Geometry: see drawing. Coordinates: mm, zero at the bounding-box minimum. A direction names the side the tool comes from. Round coordinates to 2 decimals unless told otherwise and drop trailing zeros. Loops run counter-clockwise (first coordinate to the right, second up) from the corner with the lowest first, then second, coordinate; pieces in that order, holes last.
(1) Set-up query: the marked faces 1 and 2. Return all of +Z, -Z, +X, -X, +Y, -Y with unobstructed straight access to the full face (end or side cutting, diameter ignored); none if empty.
(2) Section B-B, the plane z = 2.45. Return the cut outline in (x, y) (1 decimal).
(3) First-contact query: pin 1 Ø1.5 at (x, z) = (10, 2) entering from +Y. Flat tip, straight axial feed; report the tip coordinate or a pass-through.
(4) Section C-C, the plane x = 3. Return the cut outline in (y, z) (1 decimal).
(5) Section A-A, the plane y = 12. Return the cut outline in (x, z) (1 decimal).
(6) Material intervals for probe 1 along X at (y, z) = (20, 0.4); probe 2 along Y at (x, z) = (3.5, 2.05) (1 decimal); probe 3 along Y at (x, z) = (2.5, 2.4) (1 decimal), sorted ascending.
(7) Mould query, pull axis X, two halves, no side actions, for the marked faces 3, 4 and 5. Classes: pulls with the +X half, pulls with the -X half, needs draft (parallel to the pull), parting line crosses it, or undercut.
(8) Section D-D, the plane x = 10.5. Return the cut outline in (y, z) (1 decimal).
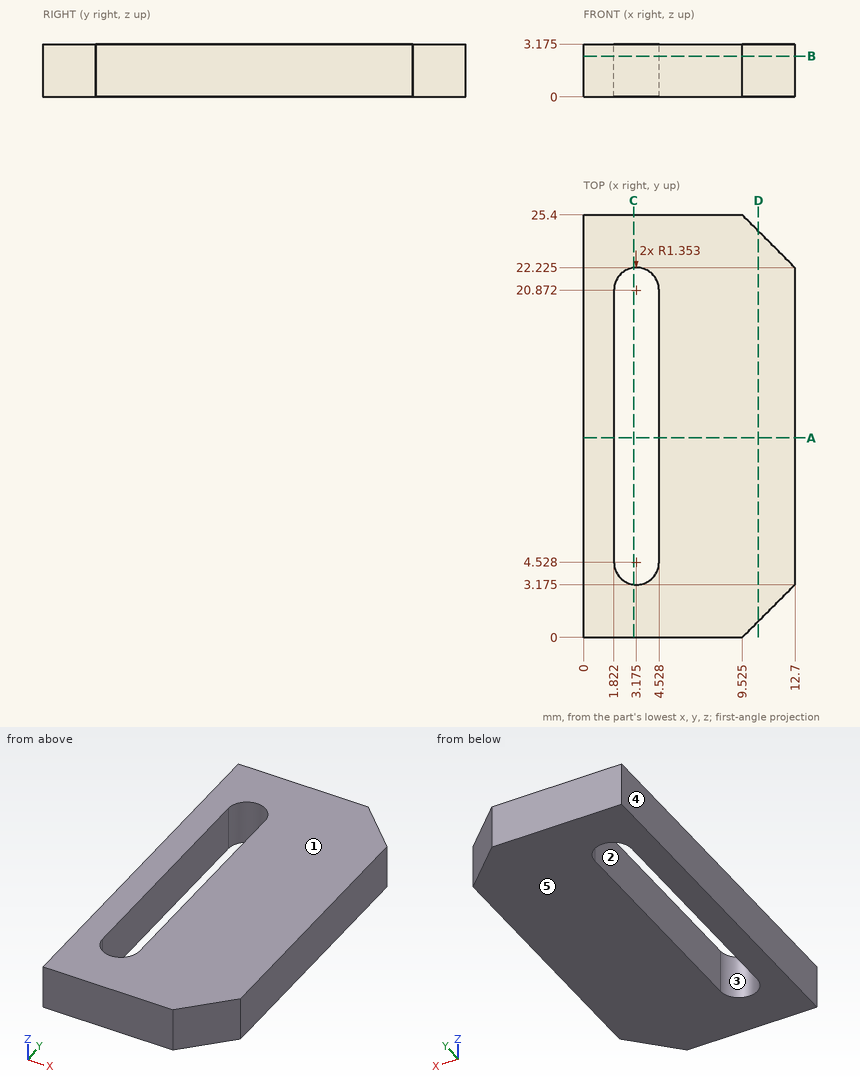
Output values:
1. face 1: +Z, +X, -X, +Y, -Y
1. face 2: +Z, -Z
2. outline: (0, 0) - (9.5, 0) - (12.7, 3.2) - (12.7, 22.2) - (9.5, 25.4) - (0, 25.4) - close; hole (1.8, 4.5) arc R1.4 ccw to (4.5, 4.5) - (4.5, 20.9) arc R1.4 ccw to (1.8, 20.9) - close
3. pin 1: stops at y = 25.4
4. outline: (0, 0) - (3.2, 0) - (3.2, 3.2) - (0, 3.2) - close; (22.2, 0) - (25.4, 0) - (25.4, 3.2) - (22.2, 3.2) - close
5. outline: (0, 0) - (1.8, 0) - (1.8, 3.2) - (0, 3.2) - close; (4.5, 0) - (12.7, 0) - (12.7, 3.2) - (4.5, 3.2) - close
6. probe 1: x = 0 to 1.82, 4.53 to 12.7
6. probe 2: y = 0 to 3.2, 22.2 to 25.4
6. probe 3: y = 0 to 3.4, 22 to 25.4
7. face 3: undercut
7. face 4: pulls with the -X half
7. face 5: needs draft
8. outline: (1, 0) - (24.4, 0) - (24.4, 3.2) - (1, 3.2) - close
